The model under review builds one solid part; all positions refer to its coordinate system, in mm. Face numbers are marked on the shaded views. A direction names the side the tool comes from. Round coordinates to 2 decimals unless told otherwise and drop trailing zeros. Loops run counter-clockwise (first coordinate to the right, second up) from the corner with the lowest first, then second, coordinate; pieces in that order, holes last. Notation, with made-up numbers: (14.25, -16.5) -> (46.25, -16.5) arc R13 cw to (46.25, 1.5) -> close; hole circle Ø5 at (31, -15.75). An arc over 180 degrees is marked (long way). Write each question's results on one line, items separated by ' | '. Start each with the question number.
Item 1: Tool access review of the marked faces 1, 2 and 3: name each direction out of +Z, -Z, +X, -X, +Y, -Y from which nothing blocks a thin tool from reaching the whole face with its end or side.
Item 2: We need section D-D (y = 37.5). Give the boundary of the cut face in (x, z), and give its area (3 significant figures).
Item 3: Clearance check with flat-ended pins moving along their axes: pin 1 Ø6 at (x, z) = (-114, 74.5) entering from -Y; pin 2 Ø3 at (x, y) = (-5, 64) entering from -Z; pin 3 Ø5 at (x, z) = (-3.5, 7.5) entering from -Y; pin 4 Ø5 at (x, z) = (-62, 610) entering from +Y. State where each tip first meets the part, or that it passes through.
Item 4: We need section A-A (x = -60). Give the boundary of the cut face in (y, z).
Item 5: We need section C-C (z = 513). Give the boundary of the cut face in (x, y), and give its area (3 significant figures).
Item 6: For L1, parallel to Z at x = -32, y = -128.5; L2, parallel to X at y = 66, z = 230; L3, parallel to Y at x = -91, z = 42.5, list the stretches that pass through material, from the lowest coordinate up. Write a range as from..to.
Item 7: Mouldability with a two-part tool opening along Z and no side actions: class the marked faces 4, 5, 6 and 7 as pulls with the +Z half, pulls with the -Z half, needs draft (parallel to the pull), parting line crosses it, or undercut.
Item 8: We need section B-B (y = -72). Give the boundary of the cut face in (x, z).
from build123d import *

# Parameters (mm, degrees)
F0_W     = 500
F0_H     = 300
F1_DEPTH = 16
F2_W     = 300
F2_H     = 100
F3_DEPTH = 266
F4_DEPTH = 16
F5_DEPTH = 250
F6_DEPTH = 16
F7_W     = 532
F7_H     = 100
F8_DEPTH = 16


with BuildPart() as f1:
    # F0 (on Top) → F1 (new body)
    with BuildSketch(Plane.XY):
        Rectangle(F0_W, F0_H)
    extrude(amount=F1_DEPTH)

    # F2 (on Right) → F3 (join, symmetric)
    with BuildSketch(Plane.YZ):
        Polygon((-150.0342194658, 600), (-150.0342194658, 100), (149.9657805342, 100), (-50.0342194658, 600), align=None)
        with Locations((-0.0342194658, 50)):
            Rectangle(F2_W, F2_H)
    extrude(amount=F3_DEPTH, both=True)

    # F4 (add): a face of the model
    f4_faces = [f1.faces().sort_by_distance(p)[0] for p in [
        (0, -100.0342194658, 600),
    ]]
    extrude(f4_faces, amount=F4_DEPTH)

    # F2 (on Right) → F5 (cut, symmetric)
    with BuildSketch(Plane.YZ):
        with Locations((-0.0342194658, 50)):
            Rectangle(F2_W, F2_H)
        Polygon((-150.0342194658, 600), (-150.0342194658, 100), (149.9657805342, 100), (-50.0342194658, 600), align=None)
    extrude(amount=F5_DEPTH, both=True, mode=Mode.SUBTRACT)

    # F0 (on Top) → F6 (join)
    with BuildSketch(Plane.XY):
        Rectangle(F0_W, F0_H)
    extrude(amount=F6_DEPTH)

    # F7 (on face) → F8 (join)
    with BuildSketch(Plane(origin=(0, 149.9657805342, 0), x_dir=(-1, 0, 0), z_dir=(0, 1, 0))):
        with Locations((0, 50)):
            Rectangle(F7_W, F7_H)
    extrude(amount=F8_DEPTH)


solid = f1.part
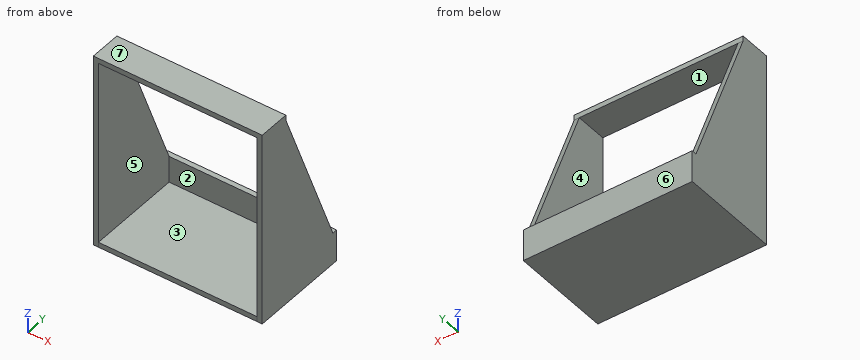
Here are the results:
1) face 1: +Y, -Y | face 2: +Z, -Y | face 3: -Y
2) outline: (-266, 0) -> (266, 0) -> (266, 381.16) -> (250, 381.16) -> (250, 16) -> (-250, 16) -> (-250, 381.16) -> (-266, 381.16) -> close | area: 20,200 mm2
3) pin 1: stops at y = 149.97 | pin 2: stops at z = 0 | pin 3: stops at y = -150 | pin 4: stops at y = -50.03
4) outline: (-150.03, 600) -> (-50.03, 600) -> (-50.03, 616) -> (-150.03, 616) -> close; (-150, 0) -> (165.97, 0) -> (165.97, 100) -> (149.97, 100) -> (149.97, 16) -> (-150, 16) -> close
5) outline: (-266, -150.03) -> (-250, -150.03) -> (-250, -15.23) -> (-266, -15.23) -> close; (250, -150.03) -> (266, -150.03) -> (266, -15.23) -> (250, -15.23) -> close | area: 4,310 mm2
6) L1: z = 0..16, 600..616 | L2: x = -266..-250, 250..266 | L3: y = 149.97..165.97
7) face 4: undercut | face 5: undercut | face 6: needs draft | face 7: pulls with the +Z half
8) outline: (-266, 0) -> (266, 0) -> (266, 616) -> (-266, 616) -> close; hole (-250, 16) -> (250, 16) -> (250, 600) -> (-250, 600) -> close
